Autodesk Inventor part; units mm, degrees
ref_plane "YZ Plane" through (0, 0, 0) normal (1, 0, 0) x (0, 1, 0)
ref_plane "XZ Plane" through (0, 0, 0) normal (0, 1, 0) x (-1, 0, 0)
ref_plane "XY Plane" through (0, 0, 0) normal (0, 0, 1) x (1, 0, 0)
sketch "Sketch1" plane through (0, 0, 0) normal (0, 0, 1) x (1, 0, 0)
  line L0 (-25, 12.5) -> (25, 12.5)
  line L1 (25, 12.5) -> (25, -12.5)
  line L2 (25, -12.5) -> (-25, -12.5)
  line L3 (-25, -12.5) -> (-25, 12.5)
  point P0 (0, 0)
  point P1 (0, 12.5)
  point P2 (-25, 0)
  dimension "d0" = 50
  dimension "d1" = 25
extrude "Extrusion1" add sketch "Sketch1" along normal blind 20
sketch "Sketch5" plane through (0, 0, 20) normal (0, 0, 1) x (1, 0, 0)
  line L0 (2.5, 8.5) -> (-12.5, 8.5) construction
  line L1 (2.5, 10.25) -> (-12.5, 10.25)
  line L2 (-12.5, 6.75) -> (2.5, 6.75)
  arc A0 (2.5, 6.75) -> (2.5, 10.25) centre (2.5, 8.5) ccw
  arc A1 (-12.5, 10.25) -> (-12.5, 6.75) centre (-12.5, 8.5) ccw
  line L3 (2.5, -6.5) -> (-12.5, -6.5) construction
  line L4 (2.5, -4.75) -> (-12.5, -4.75)
  line L5 (-12.5, -8.25) -> (2.5, -8.25)
  arc A2 (2.5, -8.25) -> (2.5, -4.75) centre (2.5, -6.5) ccw
  arc A3 (-12.5, -4.75) -> (-12.5, -8.25) centre (-12.5, -6.5) ccw
  line L6 (25, 12.5) -> (-25, 12.5)
  line L7 (-25, -12.5) -> (25, -12.5)
  line L8 (-25, 12.5) -> (-25, -12.5)
  point P0 (0, 0)
  point P1 (-5, 8.5)
  point P2 (-5, -6.5)
  dimension "d29" = 3.5
  dimension "d30" = 4
  dimension "d31" = 6
  dimension "d32" = 20
  dimension "d33" = 15
extrude "Extrusion5" cut sketch "Sketch5" against normal through all contours A2 L5 A3 L4
sketch "Sketch6" plane through (0, 0, 20) normal (0, 0, 1) x (1, 0, 0)
  line L0 (15, 0) -> (-25, 0)
  line L1 (-25, 0) -> (-25, 12.5)
  line L2 (-25, 12.5) -> (15, 12.5)
  line L3 (15, 12.5) -> (15, 0)
  line L4 (25, -12.5) -> (25, 12.5)
  line L5 (-25, 12.5) -> (-25, -12.5)
  line L6 (25, 12.5) -> (-25, 12.5)
  point P0 (0, 0)
  dimension "d36" = 10
extrude "Extrusion6" cut sketch "Sketch6" against normal through all
sketch "Sketch7" plane through (0, 0, 20) normal (0, 0, 1) x (1, 0, 0)
  line L0 (15, -12.5) -> (-25, -12.5)
  line L1 (-25, -12.5) -> (-25, 0)
  line L2 (-25, 0) -> (15, 0)
  line L3 (15, 0) -> (15, -12.5)
  line L4 (15, 12.5) -> (15, 0)
  line L5 (-25, -12.5) -> (25, -12.5)
  line L6 (-25, 0) -> (-25, -12.5)
  line L7 (15, 0) -> (-25, 0)
  point P0 (0, 0)
  point P1 (15, 2)
  point P2 (13, 0)
extrude "Extrusion7" cut sketch "Sketch7" against normal blind 12
fillet "Fillet2" radius 2 1 edges at (15, 0, 4)
mirror "Mirror1" about plane through (0, 0, 0) normal (0, 1, 0) of "Extrusion1", "Extrusion5", "Extrusion6", "Extrusion7", "Fillet2"
properties part number "0005-10-030 Activator senzor x"
CAD build for the part. Positions are in the model's coordinates, mm. A direction names the side the tool comes from. Give positions to 0.01 mm unless a question says otherwise; leave off trailing zeros. Order: outer loops, then holes, each group sorted by start corner. A loop starts at its lowest first (then second) coordinate and runs counter-clockwise, first axis right, second up.
(1) Saw through at C-C, the plane y = 5.25. Give the cut face in (x, z), then the cut area to 3 significant figures.
(2) Flat gauge pins, fed straight in: pin 1 (6 mm diameter, centred on x = -17.5, z = 11.5, fed in from +Y); pin 2 (9 mm diameter, centred on x = -3, z = 3, fed in from -Y); pin 3 (11.5 mm diameter, centred on x = -1, y = 6, fed in from +Z); pin 4 (5 mm diameter, centred on y = -10, z = 10, fed in from -X). Where does each tip first touch, or does it go through?
(3) Drill centre lines: L1, parallel to Y at x = -9.5, z = 6.75; L2, parallel to Z at x = -1, y = 0.75; L3, parallel to X at y = -10.75, z = 18.5. Where is each one in solid material? Low to high.
(4) Saw through at D-D, the plane y = 9. Give the cut face in (x, z), then the cut area to 3 significant figures.
(5) Saw through at A-A, the plane x = -8. Give the cut face in (y, z), then the cut area to 3 significant figures.
(6) Tool access for faces 1 (the flat face through (15, -3, 12)), 2 (the flat face through (-6, 0, 4)), 3 (the flat face through (-5, 8.25, 4)): list every direction of +Z, -Z, +X, -X, +Y, -Y with a clear straight run to the whole face (end or side of a thin tool).
(7) Saw through at B-B, the plane z = 5.75. Give the cut face in (x, y), then the cut area to 3 significant figures.
(8) Mould opens along X. For faces 4 (the flat face through (-5, 4, 8)), 5 (the cylindrical face through (-14.25, 6.54, 4.06)), 6 (the flat face through (-25, 6, 4)), 7 (the flat face through (-5, 4.75, 4)) say: released by +X, released by -X, zero draft, split by the parting line, or undercut.
Results found:
1. outline: (-25, 0) - (-13.72, 0) - (-13.72, 8) - (-25, 8) - close; (3.72, 0) - (25, 0) - (25, 20) - (15, 20) - (15, 8) - (3.72, 8) - close
1. area: 380 mm2
2. pin 1: passes through
2. pin 2: stops at y = 0
2. pin 3: stops at z = 8
2. pin 4: stops at x = 15
3. L1: y = 0 to 4.75, 8.25 to 12.5
3. L2: z = 0 to 8
3. L3: x = 15 to 25
4. outline: (-25, 0) - (25, 0) - (25, 20) - (15, 20) - (15, 8) - (-25, 8) - close
4. area: 520 mm2
5. outline: (0, 0) - (4.75, 0) - (4.75, 8) - (0, 8) - close; (8.25, 0) - (12.5, 0) - (12.5, 8) - (8.25, 8) - close
5. area: 72.0 mm2
6. face 1: +Z, -X, -Y
6. face 2: +Z, -Z, -X, -Y
6. face 3: +Z, -Z
7. outline: (-25, 0) - (13, 0) arc R2 cw to (15, -2) - (15, -12.5) - (25, -12.5) - (25, 12.5) - (-25, 12.5) - close; hole (-12.5, 4.75) - (2.5, 4.75) arc R1.75 ccw to (2.5, 8.25) - (-12.5, 8.25) arc R1.75 ccw to start
7. area: 689 mm2
8. face 4: zero draft
8. face 5: undercut
8. face 6: released by -X
8. face 7: undercut
